```python
from build123d import *

# Parameters (mm, degrees)
BOSS_EXTRUDE1_DEPTH = 100.35
FILLET1_R           = 10


with BuildPart() as part:
    # Sketch1 → Boss-Extrude1 (new body)
    with BuildSketch(Plane(origin=(0, 0, 0), x_dir=(1, 0, 0), z_dir=(0, 1, 0))):
        with BuildLine():
            ThreePointArc((-16.2, 0), (-13.956480682, -8.355560366), (-8.664749957, -15.2))
            Line((-8.664749957, -15.2), (8.664749957, -15.2))
            ThreePointArc((8.664749957, -15.2), (13.956480682, -8.355560366), (16.2, 0))
            ThreePointArc((16.2, 0), (13.956480682, 8.355560366), (8.664749957, 15.2))
            Line((8.664749957, 15.2), (-8.664749957, 15.2))
            ThreePointArc((-8.664749957, 15.2), (-13.956480682, 8.355560366), (-16.2, 0))
        make_face()
    extrude(amount=BOSS_EXTRUDE1_DEPTH)

    # Fillet1
    fillet1_edges = [part.edges().sort_by_distance(p)[0] for p in [
        (8.664749957, 50.175, 15.2),
        (-8.664749957, 50.175, 15.2),
        (-8.664749957, 50.175, -15.2),
        (8.664749957, 50.175, -15.2),
    ]]
    fillet(fillet1_edges, radius=FILLET1_R)


solid = part.part
```
CAD build for the part. Positions are in the model's coordinates, mm. Round coordinates to 2 decimals unless told otherwise and drop trailing zeros. Order: outer loops, then holes, each group sorted by start corner. A loop starts at its lowest first (then second) coordinate and runs counter-clockwise, first axis right, second up. Notation, with made-up numbers: (24.25, 58.25) - (50.25, 58.25) arc R25 cw to (50.25, 88.25) - close; hole circle Ø9 at (-2.75, 73.5). An arc over 180 degrees is marked (long way). Use CSV: the item, a comma, the result in double quotes. Start each with the question number.
1) Pin check, flat tips, straight feed: pin 1 Ø5 at (y, z) = (24.5, -10) entering from +X; pin 2 Ø2 at (y, z) = (14.5, 5) entering from -X; pin 3 Ø2 at (y, z) = (59, 9.5) entering from +X. Stop position of each tip, or through.
2) Saw through at A-A (y = 94.5). List the corners of the cut face in (x, z), and give its area (3 significant figures).
3) Saw through at C-C (z = 4). List the corners of the cut face in (x, y).
4) Saw through at B-B (x = -11). List the corners of the cut face in (y, z).
5) Wall check: L1, parallel to X at y = 37.5, z = 10.5; L2, parallel to X at y = 4.5, z = -13; L3, parallel to Z at x = 13, y = 38. Give the ranges that are in metal, low to high. Write a range as [from, to].
Values follow:
1,pin 1,"stops at x = 14.36"
1,pin 2,"stops at x = -15.57"
1,pin 3,"stops at x = 13.88"
2,outline,"(-16.2, 0) arc R22 ccw to (-12.6, -10.71) arc R10 ccw to (-4.26, -15.2) - (4.26, -15.2) arc R10 ccw to (12.6, -10.71) arc R22 ccw to (16.2, 0) arc R22 ccw to (12.6, 10.71) arc R10 ccw to (4.26, 15.2) - (-4.26, 15.2) arc R10 ccw to (-12.6, 10.71) arc R22 ccw to start"
2,area,"821 mm2"
3,outline,"(-15.57, 0) - (15.57, 0) - (15.57, 100.35) - (-15.57, 100.35) - close"
4,outline,"(0, -12.58) - (100.35, -12.58) - (100.35, 12.58) - (0, 12.58) - close"
5,L1,"x = [-12.74, 12.74]"
5,L2,"x = [-10.51, 10.51]"
5,L3,"z = [-10.09, 10.09]"
